```python
from build123d import *

# Parameters (mm, degrees)
BOSS_EXTRUDE1_DEPTH = 3.175
SKETCH2_W           = 3.3528
SKETCH2_H           = 6.477
SKETCH2_W_2         = 3.3782
SKETCH2_H_2         = 12.7
CUT_EXTRUDE1_DEPTH  = 4.175


with BuildPart() as part:
    # Sketch1 → Boss-Extrude1 (new body)
    with BuildSketch(Plane.XY):
        with BuildLine():
            Line((555.638244479, 111.822940833), (557.916984218, 99.326538403))
            ThreePointArc((557.916984218, 99.326538403), (326.784483289, 127.411721364), (93.98, 123.794671649))
            ThreePointArc((93.98, 123.794671649), (45.52945751, 113.491169294), (0, 93.98))
            Line((0, 93.98), (0, 106.68))
            ThreePointArc((0, 106.68), (45.466310815, 126.795024577), (93.98, 137.668))
            ThreePointArc((93.98, 137.668), (325.782502236, 142.132503557), (555.638244479, 111.822940833))
        make_face()
    extrude(amount=BOSS_EXTRUDE1_DEPTH)

    # Sketch2 → Cut-Extrude1 (cut, through all)
    with BuildSketch(Plane.XY.offset(3.175)):
        with Locations((1.6764, 97.2185)):
            Rectangle(SKETCH2_W, SKETCH2_H)
        with Locations((93.98, 122.498746884)):
            Rectangle(SKETCH2_W_2, SKETCH2_H_2)
        Polygon((183.054551015, 134.687145422), (186.429805755, 134.828179757), (186.960010022, 122.139252165), (183.584755283, 121.99821783), align=None)
        Polygon((364.577933431, 130.603714492), (367.926681813, 131.048820676), (369.239873525, 121.16904642), (365.891125143, 120.723940236), align=None)
        Polygon((298.533171127, -116.284523632), (299.081273341, -122.651898671), (295.917971315, -122.924194999), (295.369869101, -116.55681996), align=None)
        Polygon((273.590830142, 135.268456112), (276.956583497, 135.558179406), (278.045768811, 122.904971301), (274.680015455, 122.615248007), align=None)
        Polygon((456.854976279, 120.249363717), (460.178373044, 120.855391093), (461.793693389, 111.99712722), (458.470296624, 111.391099845), align=None)
        Polygon((553.540722528, 105.060688054), (556.864119293, 105.666715431), (558.657365749, 95.832721624), (555.333968984, 95.226694247), align=None)
    extrude(amount=-CUT_EXTRUDE1_DEPTH, mode=Mode.SUBTRACT)


solid = part.part
```
The model under review builds one solid part; all positions refer to its coordinate system, in mm. A direction names the side the tool comes from. Round coordinates to 2 decimals unless told otherwise and drop trailing zeros. Loops run counter-clockwise (first coordinate to the right, second up) from the corner with the lowest first, then second, coordinate; pieces in that order, holes last.
Item 1: Clearance check with a flat-ended pin moving along its axis: pin 1 Ø1.6 at (x, z) = (1, 2.5) entering from -Y. State where the tip first meets the part, or that it passes through.
Determined:
pin 1: stops at y = 100.46
Item 2: Take a section at C-C (x = 516). Write out the cut boundary in (y, z) (3 decimals).
Determined:
outline: (106.81, 0) - (119.578, 0) - (119.578, 3.175) - (106.81, 3.175) - close
Item 3: For line 1 (Y direction, x = 42.5, z = 0.7); line 2 (Y direction, x = 472, z = 0.8); line 3 (X direction, y = 99, z = 0.25), list the stretches that pass through material, from the lowest coordinate up.
Determined:
line 1: y = 112.51 to 125.8
line 2: y = 113.51 to 126.93
line 3: x = 3.35 to 9.61
Item 4: Take a section at B-B (x = 160). Write out the cut boundary in (y, z) (3 decimals).
Determined:
outline: (128.052, 0) - (142.496, 0) - (142.496, 3.175) - (128.052, 3.175) - close
Item 5: For faces 1 (the face through (413.936, 120.575, 1.565)), 2 (the face through (280, 131, 3.175)), list the 3-axis set-ups (+Z, -Z, +X, -X, +Y, -Y) from which the entire face can be reached by the end or side of a thin tool; tool diameter is ignored.
Determined:
face 1: +Z, -Z, -Y
face 2: +Z, +X, -X, +Y, -Y
Item 6: Mouldability with a two-part tool opening along X and no side actions: class faces 3 (the face through (280, 131, 0)), 4 (the face through (508.61, 108.02, 1.57)), 5 (the face through (322.54, 142.31, 1.57)), 6 (the face through (44.805, 126.576, 1.565)) as released by +X, released by -X, zero draft, split by the parting line, or undercut.
Determined:
face 3: zero draft
face 4: undercut
face 5: split by the parting line
face 6: released by -X
